CAD build for the part. Positions are in the model's coordinates, mm. A direction names the side the tool comes from. Coordinates: 2 decimals unless noted, no trailing zeros. Loops run counter-clockwise (first coordinate to the right, second up) from the corner with the lowest first, then second, coordinate; pieces in that order, holes last. Notation, with made-up numbers: (28, 84) -> (36, 84) arc R17 ccw to (36, 91) -> close; hole circle Ø10 at (-38.5, 37.25). An arc over 180 degrees is marked (long way). Write item = value, one per line. Start each with the question number.
(1) Pull direction Y, two halves, no side cores. Call faces 3 (the face through (0, 0, 3.5)), 4 (the face through (9.139, 14.334, 1.726)), 5 (the face through (0, 0, 0)): +Y half, -Y half, draft (parallel to the pull), parting line (faces both ways), or undercut.
(2) Band-saw the part on B-B (z = 10). Write the cut outline in (x, y).
(3) Drill centre lines: line 1 (Z direction, x = 2.5, y = 1); line 2 (Y direction, x = 0, z = 17.25) (3 decimals); line 3 (Y direction, x = 4.5, z = 14.5). Where is each one in solid material? Low to high. Write a range as from..to.
(4) Band-saw the part on C-C (z = 1.5). Write the cut outline in (x, y), and give its area (3 significant figures).
(5) Tool access for faces 1 (the face through (15, -5, 3.5)), 2 (the face through (-6, -8, 23)): list every direction of +Z, -Z, +X, -X, +Y, -Y with a clear straight run to the whole face (end or side of a thin tool).
(6) Band-saw the part on A-A (x = 0). Write the cut outline in (y, z), and give its area (3 significant figures).
(7) Band-saw the part on D-D (z = 13.25). Write the cut outline in (x, y), and give its area (3 significant figures).
(8) Flat gauge pins, fed straight in: P1, Ø1.5, axis at x = -12, y = -13, coming from the -Z side; P2, Ø6, axis at x = 10.5, z = 11.5, coming from the +Y side; P3, Ø8, axis at x = -1.5, y = 3.5, coming from the +Z side; P4, Ø6, axis at x = 10.5, z = 15.5, coming from the -Y side. Where does each tip first touch, or does it go through?
```python
from build123d import *

# Parameters (mm, degrees)
F1_R     = 13
F2_R     = 11.5
F5_D     = 19.4
F6_R     = 17
F7_DEPTH = 3.5
F8_R     = 3


with BuildPart() as f3:
    # F1 (on Top) → F3 section 0
    with BuildSketch(Plane.XY):
        Circle(F1_R)
    # F2 (on offset) → F3 section 1
    with BuildSketch(Plane.XY.offset(23)):
        Circle(F2_R)
    loft()

    # F5 (through all)
    with Locations(Plane(origin=(0, 0, 0), x_dir=(1, 0, 0), z_dir=(0, 0, -1))):
        with Locations((0, 0)):
            Hole(F5_D / 2)

    # F6 (on Top) → F7 (join)
    with BuildSketch(Plane.XY):
        Circle(F6_R)
    extrude(amount=F7_DEPTH)

    # F8
    f8_edges = [f3.edges().sort_by_distance(p)[0] for p in [
        (-12.771739, 0, 3.5),
    ]]
    fillet(f8_edges, radius=F8_R)


solid = f3.part
```
Findings below:
q1.face_3 = undercut
q1.face_4 = parting line
q1.face_5 = draft
q2.outline = circle Ø24.7 at (0, 0); hole circle Ø19.4 at (0, 0)
q3.line_1 = 0..3.5
q3.line_2 = -11.875..-9.7, 9.7..11.875
q3.line_3 = -11.18..-8.59, 8.59..11.18
q4.outline = circle Ø34 at (0, 0)
q4.area = 908 mm²
q5.face_1 = +Z
q5.face_2 = +Z, +X, -X, +Y, -Y
q6.outline = (-17, 0) -> (17, 0) -> (17, 3.5) -> (15.58, 3.5) arc R3 cw to (12.59, 6.3) -> (11.5, 23) -> (9.7, 23) -> (9.7, 3.5) -> (-9.7, 3.5) -> (-9.7, 23) -> (-11.5, 23) -> (-12.59, 6.3) arc R3 cw to (-15.58, 3.5) -> (-17, 3.5) -> close
q6.area = 217 mm²
q7.outline = circle Ø24.27 at (0, 0); hole circle Ø19.4 at (0, 0)
q7.area = 167 mm²
q8.P1 = 0
q8.P2 = 9.7
q8.P3 = 3.5
q8.P4 = -9.37
